from build123d import *

# Parameters (mm, degrees)
GENERALSHAPE_DEPTH           = 0.8
ADDTOLERANCE_START           = -0.8
ADDTOLERANCE_DEPTH           = 1.6
BACKPLANE_DEPTH              = 71.573791169
BACKPLANE_DEPTH_BACK         = 71.573791169
RF_W                         = 3.18
RF_H                         = 4.2
CUT_EXTRUDE1_DEPTH           = 71.587392642
FILLET1_R                    = 0.5
F_0_32_0_32_DIAMETER_HOLE1_D = 0.32
FILLET2_R                    = 0.5
FILLET3_R                    = 0.5


# Read off the part's stored shape, not the designer's step: AddTolerance
with BuildPart() as part:
    # Sketch2 → GeneralShape (new, symmetric)
    with BuildSketch(Plane(origin=(0, 0, 0), x_dir=(1, 0, 0), z_dir=(0, 1, 0))):
        Polygon((47.25, 46.4), (34.5, 46.4), (34.5, 50), (-34.5, 50), (-34.5, 46.4), (-47.25, 46.4), (-47.25, 41.5), (-50, 41.5), (-50, -38.9), (-41.5, -47.4), (41.5, -47.4), (50, -38.9), (50, 41.5), (47.25, 41.5), align=None)
    extrude(amount=GENERALSHAPE_DEPTH, both=True)

    # AddTolerance outline → AddTolerance (cut)
    with BuildSketch(Plane(origin=(0, 0, 0), x_dir=(1, 0, 0), z_dir=(0, 1, 0)).offset(ADDTOLERANCE_START)):
        Polygon((49.9, 41.4), (49.9, -39), (50, -38.9), (50, 41.5), (47.25, 41.5), (47.25, 46.4), (34.5, 46.4), (34.5, 50), (-34.5, 50), (-34.5, 46.4), (-47.25, 46.4), (-47.25, 41.5), (-50, 41.5), (-50, -38.9), (-49.9, -39), (-49.9, 41.4), (-47.15, 41.4), (-47.15, 46.3), (-34.4, 46.3), (-34.4, 49.9), (34.4, 49.9), (34.4, 46.3), (47.15, 46.3), (47.15, 41.4), align=None)
    extrude(amount=ADDTOLERANCE_DEPTH, mode=Mode.SUBTRACT)

    # Sketch4 → Backplane (cut, two sides: drawn at the far end of the back side and taken through both)
    with BuildSketch(Plane(origin=(0, 0, 0), x_dir=(1, 0, 0), z_dir=(0, 1, 0)).offset(-BACKPLANE_DEPTH_BACK)):
        with BuildLine():
            Line((41.5, -47.4), (44.1, -44.8))
            Line((44.1, -44.8), (41.232050808, -44.8))
            ThreePointArc((41.232050808, -44.8), (39.5, -43.8), (37.767949192, -44.8))
            Line((37.767949192, -44.8), (18.232050808, -44.8))
            ThreePointArc((18.232050808, -44.8), (16.5, -43.8), (14.767949192, -44.8))
            Line((14.767949192, -44.8), (-14.767949192, -44.8))
            ThreePointArc((-14.767949192, -44.8), (-16.5, -43.8), (-18.232050808, -44.8))
            Line((-18.232050808, -44.8), (-37.767949192, -44.8))
            ThreePointArc((-37.767949192, -44.8), (-39.5, -43.8), (-41.232050808, -44.8))
            Line((-41.232050808, -44.8), (-44.1, -44.8))
            Line((-44.1, -44.8), (-41.5, -47.4))
            Line((-41.5, -47.4), (41.5, -47.4))
        make_face()
    extrude(amount=BACKPLANE_DEPTH + BACKPLANE_DEPTH_BACK, mode=Mode.SUBTRACT)

    # RF → Cut-Extrude1 (cut, through all)
    with BuildSketch(Plane(origin=(0, 0.8, 0), x_dir=(1, 0, 0), z_dir=(0, 1, 0))):
        with Locations((-22, -38.7)):
            Rectangle(RF_W, RF_H)
        with Locations((-28, -38.7)):
            Rectangle(RF_W, RF_H)
        with Locations((-34, -38.7)):
            Rectangle(RF_W, RF_H)
        with BuildLine():
            Line((-18.232050808, -40.8), (-20.41, -40.8))
            Line((-20.41, -40.8), (-23.59, -40.8))
            Line((-23.59, -40.8), (-26.41, -40.8))
            Line((-26.41, -40.8), (-29.59, -40.8))
            Line((-29.59, -40.8), (-32.41, -40.8))
            Line((-32.41, -40.8), (-35.59, -40.8))
            Line((-35.59, -40.8), (-37.767949192, -40.8))
            Line((-37.767949192, -40.8), (-37.767949192, -43.8))
            Line((-37.767949192, -43.8), (-39.5, -43.8))
            ThreePointArc((-39.5, -43.8), (-38.5, -44.067949192), (-37.767949192, -44.8))
            Line((-37.767949192, -44.8), (-18.232050808, -44.8))
            ThreePointArc((-18.232050808, -44.8), (-17.5, -44.067949192), (-16.5, -43.8))
            Line((-16.5, -43.8), (-18.232050808, -43.8))
            Line((-18.232050808, -43.8), (-18.232050808, -40.8))
        make_face()
    extrude(amount=-CUT_EXTRUDE1_DEPTH, mode=Mode.SUBTRACT)

    # Fillet1
    fillet1_edges = [part.edges().sort_by_distance(p)[0] for p in [
        (-23.59, 0, 36.6),
        (-20.41, 0, 36.6),
        (-18.232050808, 0, 40.8),
        (-18.232050808, 0, 43.8),
        (-37.767949192, 0, 43.8),
        (-37.767949192, 0, 40.8),
        (-35.59, 0, 36.6),
        (-32.41, 0, 36.6),
        (-29.59, 0, 36.6),
        (-26.41, 0, 36.6),
    ]]
    fillet(fillet1_edges, radius=FILLET1_R)

    # Ø0.32 (0.32) Diameter Hole1 (through all)
    with Locations(Plane(origin=(0, 0.8, 0), x_dir=(1, 0, 0), z_dir=(0, 1, 0))):
        with Locations((-20.41, -36.6), (-23.59, -36.6), (-26.41, -36.6), (-29.59, -36.6), (-32.41, -36.6), (-35.59, -36.6)):
            Hole(F_0_32_0_32_DIAMETER_HOLE1_D / 2)

    # Fillet2
    fillet2_edges = [part.edges().sort_by_distance(p)[0] for p in [
        (47.15, 0, -41.4),
        (47.15, 0, -46.3),
        (34.4, 0, -46.3),
        (-34.4, 0, -46.3),
        (-47.15, 0, -46.3),
        (-47.15, 0, -41.4),
    ]]
    fillet(fillet2_edges, radius=FILLET2_R)

    # Fillet3
    fillet3_edges = [part.edges().sort_by_distance(p)[0] for p in [
        (49.9, 0, -41.4),
        (34.4, 0, -49.9),
        (-34.4, 0, -49.9),
        (-49.9, 0, -41.4),
    ]]
    fillet(fillet3_edges, radius=FILLET3_R)


solid = part.part
The model under review builds one solid part; all positions refer to its coordinate system, in mm. Coordinates: 2 decimals unless noted, no trailing zeros. Answer in a Markdown table with one row per item.
1. Wall thickness on probe 1 along Z at (x, y) = (36.5, -0.7); probe 2 along Z at (x, y) = (-34, 0.6); probe 3 along X at (y, z) = (0.7, -43.5): over which ranges is each line inside the solid? List them lowest first. Write a range as [from, to].
Answers below:
| item | result |
|---|---|
| probe 1 | z = [-46.3, 44.8] |
| probe 2 | z = [-49.89, 36.6] |
| probe 3 | x = [-47.15, 47.15] |
2. We need section A-A, the plane y = -0.3. Give the number of separate pieces and of enclosed holes in the cut face, and give its area (3 significant figures).
Answers below:
| item | result |
|---|---|
| separate pieces | 1 |
| enclosed holes | 6 |
| area | 9,150 mm^2 |
3. Clearance check with flat-ended pins moving along their axes: pin 1 Ø0.5 at (x, y) = (48.5, 0) entering from -Z; pin 2 Ø0.8 at (x, y) = (43, 0) entering from -Z; pin 3 Ø0.8 at (x, y) = (-19.5, 0.5) entering from +Z. State where each tip first meets the part, or that it passes through.
Answers below:
| item | result |
|---|---|
| pin 1 | stops at z = -41.4 |
| pin 2 | stops at z = -46.3 |
| pin 3 | stops at z = 40.8 |
